Geometry check sheet. Reference: the model listing, model coordinates, mm. Round coordinates to 2 decimals unless told otherwise and drop trailing zeros. Order: outer loops, then holes, each group sorted by start corner. A loop starts at its lowest first (then second) coordinate and runs counter-clockwise, first axis right, second up.
(1) Cross-section at B-B on z = -3. Enter the section's corners in (x, y).
(2) Thickness scan on L1, parallel to X at y = 1, z = -3; L2, parallel to Z at x = 14.5, y = 1.5; L3, parallel to Z at x = 13, y = 0.6. Record the ranges inside material, lowest first.
(3) Draft check along Z on faces 1 (the face through (14.45, 0.79, -55.57)), 2 (the face through (10, 1, 0)), 3 (the face through (20, 1, -30)), 4 (the face through (10, 1, -60)). Enter one of: pulls with the +Z half, pulls with the -Z half, needs draft (parallel to the pull), parting line crosses it, or undercut.
(4) Cross-section at A-A on x = 14. Enter the section's corners in (y, z).
(5) Gauge pin test, flat end, axial feed: P1, Ø1.8, axis at x = 14, z = -3, coming from the +Y side. Record the tip position at first contact, or that the pin passes through.
from build123d import *

# Parameters (mm, degrees)
SKETCH1_W       = 20
SKETCH1_H       = 60
SKETCH1_R       = 1.5
PCB_BOARD_DEPTH = 1.6


with BuildPart() as part:
    # Sketch1 → pcb_board (new body)
    with BuildSketch(Plane(origin=(0, 0, 0), x_dir=(1, 0, 0), z_dir=(0, 1, 0))):
        with Locations((10, 30)):
            Rectangle(SKETCH1_W, SKETCH1_H)
        with Locations(Location((14, 3, 0), (0, 0, 270))):
            Circle(SKETCH1_R, mode=Mode.SUBTRACT)
        with Locations(Location((14, 57, 0), (0, 0, 270))):
            Circle(SKETCH1_R, mode=Mode.SUBTRACT)
    extrude(amount=PCB_BOARD_DEPTH)


solid = part.part
Found:
1. outline: (0, 0) - (12.5, 0) - (12.5, 1.6) - (0, 1.6) - close; (15.5, 0) - (20, 0) - (20, 1.6) - (15.5, 1.6) - close
2. L1: x = 0 to 12.5, 15.5 to 20
2. L2: z = -60 to -58.41, -55.59 to -4.41, -1.59 to 0
2. L3: z = -60 to -58.12, -55.88 to -4.12, -1.88 to 0
3. face 1: undercut
3. face 2: pulls with the +Z half
3. face 3: needs draft
3. face 4: pulls with the -Z half
4. outline: (0, -60) - (1.6, -60) - (1.6, -58.5) - (0, -58.5) - close; (0, -55.5) - (1.6, -55.5) - (1.6, -4.5) - (0, -4.5) - close; (0, -1.5) - (1.6, -1.5) - (1.6, 0) - (0, 0) - close
5. P1: passes through
